from build123d import *

# Parameters (mm, degrees)
SKETCH1_W           = 6.35
SKETCH1_H           = 9
SKETCH1_R           = 1.5875
BOSS_EXTRUDE1_DEPTH = 30
SKETCH2_R           = 1.59
CUT_EXTRUDE1_DEPTH  = 30


with BuildPart() as part:
    # Sketch1 → Boss-Extrude1 (new body)
    with BuildSketch(Plane.XY):
        with Locations((3.175, -4.5)):
            Rectangle(SKETCH1_W, SKETCH1_H)
        with Locations((3.175, -6.5)):
            Circle(SKETCH1_R, mode=Mode.SUBTRACT)
    extrude(amount=BOSS_EXTRUDE1_DEPTH)

    # Sketch2 → Cut-Extrude1 (cut)
    with BuildSketch(Plane(origin=(0, 0, 0), x_dir=(0, 0, -1), z_dir=(1, 0, 0))):
        with Locations((-21.35, -3)):
            Circle(SKETCH2_R)
        with Locations((-8.65, -3)):
            Circle(SKETCH2_R)
    extrude(amount=CUT_EXTRUDE1_DEPTH, mode=Mode.SUBTRACT)


solid = part.part
The model under review builds one solid part; all positions refer to its coordinate system, in mm. Coordinates: 2 decimals unless noted, no trailing zeros. Loops run counter-clockwise (first coordinate to the right, second up) from the corner with the lowest first, then second, coordinate; pieces in that order, holes last. Notation, with made-up numbers: M -40,22 L -26,22 A17 cw -26,50 Z; hole C 83,-18 d1. An arc over 180 degrees is marked long. Put each result on its own line as item: value. Start each with the question number.
Q1. Add section C-C (x = 3). Write out the cut boundary in (y, z), and give its area (3 significant figures).
Q2. Add section A-A (z = 8.65). Count the separate pieces of the cut face and the enclosed holes in it, and give its area (3 significant figures).
Q3. Wall thickness on line 1 (Z direction, x = 4, y = -3); line 2 (Y direction, x = 3.25, z = 14.75); line 3 (Y direction, x = 4, z = 8.65): over which ranges is each line inside the solid? List them lowest first.
Q4. Add section D-D (y = -3). Write out the cut boundary in (x, z), and give its area (3 significant figures).
Q5. Add section B-B (y = -6.5). Write out the cut boundary in (x, z).
Q6. The part is to be moulded in two halves that separate along Y. For faces 1 (the flat face through (6.35, -5, 15)), 2 (the cylindrical face through (3.13, -3.61, 19.88)), 3 (the flat face through (3, -9, 15)), say which applies: +Y half, -Y half, draft (parallel to the pull), parting line (faces both ways), or undercut.
Answers:
1. outline: M -9,0 L -8.08,0 L -8.08,30 L -9,30 Z; M -4.92,0 L 0,0 L 0,30 L -4.92,30 Z; hole C -3,8.65 d3.18; hole C -3,21.35 d3.18
1. area: 159 mm^2
2. separate pieces: 2
2. enclosed holes: 1
2. area: 29.0 mm^2
3. line 1: z = 0 to 7.06, 10.24 to 19.76, 22.94 to 30
3. line 2: y = -9 to -8.09, -4.91 to 0
3. line 3: y = -9 to -7.86, -5.14 to -4.59, -1.41 to 0
4. outline: M 0,0 L 6.35,0 L 6.35,7.06 L 0,7.06 Z; M 0,10.24 L 6.35,10.24 L 6.35,19.76 L 0,19.76 Z; M 0,22.94 L 6.35,22.94 L 6.35,30 L 0,30 Z
4. area: 150 mm^2
5. outline: M 0,0 L 1.59,0 L 1.59,30 L 0,30 Z; M 4.76,0 L 6.35,0 L 6.35,30 L 4.76,30 Z
6. face 1: draft
6. face 2: undercut
6. face 3: -Y half
